from build123d import *

# Parameters (mm, degrees)
F0_W     = 40
F0_H     = 26
F1_DEPTH = 15
F2_R     = 8.5
F2_R_2   = 2
F3_DEPTH = 15.001


with BuildPart() as f1:
    # F0 (on Top) → F1 (new body)
    with BuildSketch(Plane.XY):
        Rectangle(F0_W, F0_H)
    extrude(amount=F1_DEPTH)

    # F2 (on face) → F3 (cut, through all)
    with BuildSketch(Plane.XY.offset(15)):
        Circle(F2_R)
        with Locations((-16, 9)):
            Circle(F2_R_2)
        with Locations((-16, -9)):
            Circle(F2_R_2)
        with Locations((16, 9)):
            Circle(F2_R_2)
        with Locations((16, -9)):
            Circle(F2_R_2)
    extrude(amount=-F3_DEPTH, mode=Mode.SUBTRACT)


solid = f1.part
Model file for the job. Use its own axes, mm. Round coordinates to 2 decimals unless told otherwise and drop trailing zeros. Loops run counter-clockwise (first coordinate to the right, second up) from the corner with the lowest first, then second, coordinate; pieces in that order, holes last. Notation, with made-up numbers: (69, -27) - (108, -27) arc R17 ccw to (108, -16) - close; hole circle Ø3 at (-14, 22). An arc over 180 degrees is marked (long way). Write each question's results on one line, items separated by ' | '.
(1) Wall check: L1, parallel to Y at x = 0, z = 6.75; L2, parallel to X at y = 10.75, z = 10; L3, parallel to X at y = -7.5, z = 5.5. Give the ranges that are in metal, low to high.
Answer below:
L1: y = -13 to -8.5, 8.5 to 13 | L2: x = -20 to -16.97, -15.03 to 15.03, 16.97 to 20 | L3: x = -20 to -17.32, -14.68 to -4, 4 to 14.68, 17.32 to 20
(2) Saw through at C-C, the plane y = 3.25. List the corners of the cut face in (x, z), then the cut area to 3 significant figures.
Answer below:
outline: (-20, 0) - (-7.85, 0) - (-7.85, 15) - (-20, 15) - close; (7.85, 0) - (20, 0) - (20, 15) - (7.85, 15) - close | area: 364 mm^2
(3) Saw through at A-A, the plane x = 16. List the corners of the cut face in (y, z).
Answer below:
outline: (-13, 0) - (-11, 0) - (-11, 15) - (-13, 15) - close; (-7, 0) - (7, 0) - (7, 15) - (-7, 15) - close; (11, 0) - (13, 0) - (13, 15) - (11, 15) - close
(4) Saw through at D-D, the plane x = 0. List the corners of the cut face in (y, z), then the cut area to 3 significant figures.
Answer below:
outline: (-13, 0) - (-8.5, 0) - (-8.5, 15) - (-13, 15) - close; (8.5, 0) - (13, 0) - (13, 15) - (8.5, 15) - close | area: 135 mm^2
(5) Mould opens along Y. For faces 1 (the cylindrical face through (-17.474, 10.352, 7.605)), 2 (the flat face through (-20, 0, 7)), 3 (the flat face through (0, -13, 7)) say: released by +Y, released by -Y, zero draft, split by the parting line, or undercut.
Answer below:
face 1: undercut | face 2: zero draft | face 3: released by -Y
(6) Saw through at B-B, the plane z = 9. List the corners of the cut face in (x, y), then the cut area to 3 significant figures.
Answer below:
outline: (-20, -13) - (20, -13) - (20, 13) - (-20, 13) - close; hole circle Ø4 at (-16, -9); hole circle Ø4 at (-16, 9); hole circle Ø17 at (0, 0); hole circle Ø4 at (16, -9); hole circle Ø4 at (16, 9) | area: 763 mm^2
